Source: CAD feature listing. Evaluate the final solid. Frame: model axes, mm. A direction names the side the tool comes from. Give positions to 0.01 mm unless a question says otherwise; leave off trailing zeros. Write each loop counter-clockwise with the first axis right and the second up, starting at its lowest first coordinate (ties: lowest second). Pieces come first, ordered by that corner, then holes. Notation, with made-up numbers: (12, 17.5) -> (19, 17.5) arc R18 cw to (19, 46.5) -> close; hole circle Ø3 at (69.5, 19). An arc over 180 degrees is marked (long way). Write item = value, one per line.
from build123d import *

# Parameters (mm, degrees)
F0_R     = 23.385551
F1_DEPTH = 127
F2_R     = 16.56705
F3_DEPTH = 76.2


with BuildPart() as f1:
    # F0 (on Top) → F1 (new body)
    with BuildSketch(Plane.XY):
        Circle(F0_R)
    extrude(amount=F1_DEPTH)


with BuildPart() as f3:
    # F2 (on Top) → F3 (new body)
    with BuildSketch(Plane.XY):
        Circle(F2_R)
    extrude(amount=F3_DEPTH)


with BuildPart() as f1_1:
    add(f1.part)

    # F4: cut F3
    add(f3.part, mode=Mode.SUBTRACT)


solid = f1_1.part
(1) Section query A-A (y = 0). Return loops of the section in (x, z), plus the area to 3 significant figures.
Values follow:
outline = (-23.39, 0) -> (-16.57, 0) -> (-16.57, 76.2) -> (16.57, 76.2) -> (16.57, 0) -> (23.39, 0) -> (23.39, 127) -> (-23.39, 127) -> close
area = 3,420 mm2
(2) Material intervals for line 1 (Y direction, x = 0, z = 25); line 2 (Z direction, x = -5.5, y = 12.5); line 3 (Y direction, x = 4.5, z = 54), sorted ascending.
Values follow:
line_1 = -23.39 to -16.57, 16.57 to 23.39
line_2 = 76.2 to 127
line_3 = -22.95 to -15.94, 15.94 to 22.95
(3) Section query D-D (x = 20.5). Return loops of the section in (y, z).
Values follow:
outline = (-11.25, 0) -> (11.25, 0) -> (11.25, 127) -> (-11.25, 127) -> close
(4) Section query C-C (z = 68). Return loops of the section in (x, y).
Values follow:
outline = circle Ø46.77 at (0, 0); hole circle Ø33.13 at (0, 0)
(5) Access query for faces 4 (the face through (0, 0, 76.2)), 5 (the face through (-16, -5, 0)). Directions: +Z, -Z, +X, -X, +Y, -Y. A direction counts if a zero-diameter tool reaches every point of the face in a straight line with its end or side. Return the directions, or none.
Values follow:
face_4 = -Z
face_5 = -Z, +X, -X, +Y, -Y
(6) First-contact query: pin 1 (4 mm diameter, centred on x = -11, z = 23, fed in from +Y); pin 2 (5 mm diameter, centred on y = -8, z = 44, fed in from +X); pin 3 (1.5 mm diameter, centred on y = 4, z = 73.5, fed in from -X). Flat tips, straight axial feed; report the tip coordinate or a pass-through.
Values follow:
pin_1 = 21.58
pin_2 = 22.73
pin_3 = -23.16
(7) Pull-direction query (X, two-part tool) for faces 1 (the face through (0, 0, 127)), 2 (the face through (-2.157, 16.426, 37.567)), 3 (the face through (-23.363, 1.028, 62.611)); classes: pulls with the +X half, pulls with the -X half, needs draft (parallel to the pull), parting line crosses it, or undercut.
Values follow:
face_1 = needs draft
face_2 = undercut
face_3 = parting line crosses it
